Autodesk Fusion 360 part; units mm, degrees
sketch "Sketch1" plane through (0, 0, 0) normal (0, 0, 1) x (1, 0, 0)
  line L0 (0, 101) -> (134.5, 101)
  line L1 (134.5, 101) -> (134.5, 0)
  line L2 (134.5, 0) -> (205, 0)
  line L3 (205, 0) -> (205, 167.5)
  line L4 (205, 167.5) -> (0, 167.5)
  line L5 (0, 167.5) -> (0, 101)
  line L6 (-134.5, 101) -> (-134.5, 0)
  line L7 (-205, 0) -> (-205, 167.5)
  line L8 (-205, 167.5) -> (0, 167.5)
  line L9 (0, 101) -> (-134.5, 101)
  line L10 (0, 167.5) -> (0, 101)
  line L11 (-134.5, 0) -> (-205, 0)
  line L12 (134.5, -101) -> (134.5, 0)
  line L13 (205, -167.5) -> (0, -167.5)
  line L14 (0, -167.5) -> (0, -101)
  line L15 (0, -101) -> (-134.5, -101)
  line L16 (-134.5, 0) -> (-205, 0)
  line L17 (205, 0) -> (205, -167.5)
  line L18 (-205, 0) -> (-205, -167.5)
  line L19 (-205, -167.5) -> (0, -167.5)
  line L20 (-134.5, -101) -> (-134.5, 0)
  line L21 (0, -167.5) -> (0, -101)
  line L22 (0, -101) -> (134.5, -101)
  line L23 (134.5, 0) -> (205, 0)
  dimension "d26" = 101
  dimension "d27" = 134.5
  dimension "d28" = 101
  dimension "d29" = 70.5
  dimension "d30" = 167.5
  dimension "d31" = 205
  dimension "d32" = 66.5
extrude "Extrude4" add sketch "Sketch1" along normal blind 2 contours L0 L1 L2 L3 L4 L5 L10 L23 | L5 L6 L7 L8 L9 L10 L11 L16 | L2 L12 L13 L14 L17 L21 L22 L23 | L11 L14 L15 L16 L18 L19 L20 L21
chamfer "Chamfer2" distance 1 angle 45 4 edges at (0, 101, 2) (-134.5, 0, 2) (0, -101, 2) (134.5, 0, 2)
fillet "Fillet1" radius 2.5 4 edges at (205, -167.5, 1) (205, 167.5, 1) (-205, -167.5, 1) (-205, 167.5, 1)
The listing builds one solid part. Answer for the finished solid, in the listing's coordinates (mm). Give positions to 0.01 mm unless a question says otherwise; leave off trailing zeros. Order: outer loops, then holes, each group sorted by start corner. A loop starts at its lowest first (then second) coordinate and runs counter-clockwise, first axis right, second up. Notation, with made-up numbers: (-6, 40) - (20, 40) arc R27 cw to (20, 78) - close; hole circle Ø11 at (54.5, 78.5). An arc over 180 degrees is marked (long way). Answer as CSV lines item,"result".
Q1. Straight lines are drawn through the part: L1, parallel to Y at x = 133.5, z = 0.95; L2, parallel to Y at x = 51, z = 1.05; L3, parallel to X at y = -78, z = 0.7. For each, find the intervals that lie inside material, in ascending order.
Answer key:
L1,"y = -167.5 to -101, 101 to 167.5"
L2,"y = -167.5 to -101.05, 101.05 to 167.5"
L3,"x = -205 to -134.5, 134.5 to 205"
Q2. A cutting plane is placed at B-B, the plane z = 1.5. Determine the outline of the cut face in (x, y), and give its area (3 significant figures).
Answer key:
outline,"(-205, -165) arc R2.5 ccw to (-202.5, -167.5) - (202.5, -167.5) arc R2.5 ccw to (205, -165) - (205, 165) arc R2.5 ccw to (202.5, 167.5) - (-202.5, 167.5) arc R2.5 ccw to (-205, 165) - close; hole (-135, -101.5) - (135, -101.5) - (135, 101.5) - (-135, 101.5) - close"
area,"82,500 mm^2"
Q3. A cutting plane is placed at A-A, the plane x = 3. Determine the outline of the cut face in (y, z).
Answer key:
outline,"(-167.5, 0) - (-101, 0) - (-101, 1) - (-102, 2) - (-167.5, 2) - close; (101, 0) - (167.5, 0) - (167.5, 2) - (102, 2) - (101, 1) - close"
Q4. A cutting plane is placed at C-C, the plane y = 68. Determine the outline of the cut face in (x, z), and give its area (3 significant figures).
Answer key:
outline,"(-205, 0) - (-134.5, 0) - (-134.5, 1) - (-135.5, 2) - (-205, 2) - close; (134.5, 0) - (205, 0) - (205, 2) - (135.5, 2) - (134.5, 1) - close"
area,"281 mm^2"
